Autodesk Inventor part; units mm, degrees
ref_plane "YZ Plane" through (0, 0, 0) normal (1, 0, 0) x (0, 1, 0)
ref_plane "XZ Plane" through (0, 0, 0) normal (0, 1, 0) x (-1, 0, 0)
ref_plane "XY Plane" through (0, 0, 0) normal (0, 0, 1) x (1, 0, 0)
sketch "스케치3" plane through (0, 0, 0) normal (0, 1, 0) x (-1, 0, 0)
  line L0 (34.9919, -14.4941) -> (14.4941, -34.9919)
  line L1 (14.4941, -34.9919) -> (-14.4941, -34.9919)
  line L2 (-14.4941, -34.9919) -> (-34.9919, -14.4941)
  line L3 (-34.9919, -14.4941) -> (-34.9919, 14.4941)
  line L4 (-34.9919, 14.4941) -> (-14.4941, 34.9919)
  line L5 (-14.4941, 34.9919) -> (14.4941, 34.9919)
  line L6 (14.4941, 34.9919) -> (34.9919, 14.4941)
  line L7 (34.9919, 14.4941) -> (34.9919, -14.4941)
  line L8 (32.5919, -13.5) -> (13.5, -32.5919)
  line L9 (13.5, -32.5919) -> (-13.5, -32.5919)
  line L10 (-13.5, -32.5919) -> (-32.5919, -13.5)
  line L11 (-32.5919, -13.5) -> (-32.5919, 13.5)
  line L12 (-32.5919, 13.5) -> (-13.5, 32.5919)
  line L13 (-13.5, 32.5919) -> (13.5, 32.5919)
  line L14 (13.5, 32.5919) -> (32.5919, 13.5)
  line L15 (32.5919, 13.5) -> (32.5919, -13.5)
  point P0 (0, 0)
  point P1 (0, 0)
  point P2 (0, 0)
  point P3 (0, 0)
  dimension "d43" = 27
  dimension "d44" = 2.4
extrude "돌출2" add sketch "스케치3" along normal blind 3.4 contours L0 L1 L2 L3 L4 L5 L6 L7 | L8 L9 L10 L11 L12 L13 L14 L15
sketch "스케치4" plane through (0, 3.4, 0) normal (0, 1, 0) x (1, 0, 0)
  line L0 (13.5, -32.5919) -> (-13.5, -32.5919)
  line L1 (-13.5, -32.5919) -> (-32.5919, -13.5)
  line L2 (-32.5919, -13.5) -> (-32.5919, 13.5)
  line L3 (-32.5919, 13.5) -> (-13.5, 32.5919)
  line L4 (-13.5, 32.5919) -> (13.5, 32.5919)
  line L5 (13.5, 32.5919) -> (32.5919, 13.5)
  line L6 (32.5919, 13.5) -> (32.5919, -13.5)
  line L7 (32.5919, -13.5) -> (13.5, -32.5919)
  line L8 (-13.9971, 33.7919) -> (13.9971, 33.7919)
  line L9 (13.9971, 33.7919) -> (33.7919, 13.9971)
  line L10 (33.7919, 13.9971) -> (33.7919, -13.9971)
  line L11 (33.7919, -13.9971) -> (13.9971, -33.7919)
  line L12 (13.9971, -33.7919) -> (-13.9971, -33.7919)
  line L13 (-13.9971, -33.7919) -> (-33.7919, -13.9971)
  line L14 (-33.7919, -13.9971) -> (-33.7919, 13.9971)
  line L15 (-33.7919, 13.9971) -> (-13.9971, 33.7919)
  line L16 (-13.1686, 31.7919) -> (13.1686, 31.7919)
  line L17 (13.1686, 31.7919) -> (31.7919, 13.1686)
  line L18 (31.7919, 13.1686) -> (31.7919, -13.1686)
  line L19 (31.7919, -13.1686) -> (13.1686, -31.7919)
  line L20 (13.1686, -31.7919) -> (-13.1686, -31.7919)
  line L21 (-13.1686, -31.7919) -> (-31.7919, -13.1686)
  line L22 (-31.7919, -13.1686) -> (-31.7919, 13.1686)
  line L23 (-31.7919, 13.1686) -> (-13.1686, 31.7919)
  point P0 (0, 0)
  point P1 (0, 0)
  point P2 (0, 0)
  point P3 (0, 0)
  dimension "d7" = 27
  dimension "d42" = 1.2
  dimension "d45" = 0.8
extrude "돌출3" cut sketch "스케치4" against normal blind 1.2 contours L0 L1 L2 L3 L4 L5 L6 L7 | L8 L9 L10 L11 L12 L13 L14 L15 | L16 L17 L18 L19 L20 L21 L22 L23
sketch "스케치5" plane through (0, 0, 0) normal (0, -1, 0) x (1, 0, 0)
  line L0 (10, 2.5) -> (20, 2.5)
  line L1 (20, 2.5) -> (20, -2.5)
  line L2 (20, -2.5) -> (10, -2.5)
  line L3 (10, -2.5) -> (10, 2.5)
  line L4 (10, 2.5) -> (20, -2.5) construction
  line L5 (20, 2.5) -> (10, -2.5) construction
  line L6 (-20, 2.5) -> (-10, 2.5)
  line L7 (-10, 2.5) -> (-10, -2.5)
  line L8 (-10, -2.5) -> (-20, -2.5)
  line L9 (-20, -2.5) -> (-20, 2.5)
  line L10 (-20, 2.5) -> (-10, -2.5) construction
  line L11 (-10, 2.5) -> (-20, -2.5) construction
  point P0 (0, 0)
  point P1 (15, 0)
  point P2 (-15, 0)
  dimension "d11" = 10
  dimension "d12" = 5
  dimension "d13" = 10
  dimension "d16" = 30
extrude "돌출4" add sketch "스케치5" along normal blind 10
sketch "스케치6" plane through (-10, 0, -2.5) normal (0, 0, -1) x (-1, 0, 0)
  circle A0 centre (5, -10) radius 5
  circle A1 centre (-25, -10) radius 5
  line L0 (-20, -10) -> (-30, -10)
  line L1 (10, -10) -> (0, -10)
  point P0 (-10, 0)
  dimension "d23" = 10
  dimension "d24" = 10
extrude "돌출5" add sketch "스케치6" against normal blind 5
sketch "스케치7" plane through (-10, 0, -2.5) normal (0, 0, -1) x (-1, 0, 0)
  circle A0 centre (5, -10) radius 1.25
  line L0 (10, 0) -> (10, -10)
  line L1 (0, 0) -> (10, 0)
  line L2 (4.7788, 0) -> (0, 0)
  circle A1 centre (-25, -10) radius 1.25
  point P0 (-10, 0)
  dimension "d27" = 2.5
  dimension "d28" = 5
  dimension "d31" = 30
extrude "돌출6" cut sketch "스케치7" against normal blind 5
sketch "스케치8" plane through (0, 0, 0) normal (0, -1, 0) x (1, 0, 0)
  circle A0 centre (0, -17.3205) radius 1.25
  line L0 (-10, 2.5) -> (-10, -2.5)
  point P0 (0, 0)
  point P1 (-10, 0)
  dimension "d38" = 2.5
  dimension "d39" = 17.3205
extrude "돌출7" cut sketch "스케치8" against normal blind 5
sketch "스케치9" plane through (0, 2.2, 0) normal (0, 1, 0) x (1, 0, 0)
  line L0 (-13.1686, 31.7919) -> (13.1686, 31.7919)
  line L1 (13.1686, 31.7919) -> (31.7919, 13.1686)
  line L2 (31.7919, 13.1686) -> (31.7919, -13.1686)
  line L3 (31.7919, -13.1686) -> (13.1686, -31.7919)
  line L4 (13.1686, -31.7919) -> (-13.1686, -31.7919)
  line L5 (-13.1686, -31.7919) -> (-31.7919, -13.1686)
  line L6 (-31.7919, -13.1686) -> (-31.7919, 13.1686)
  line L7 (-31.7919, 13.1686) -> (-13.1686, 31.7919)
  line L8 (-13.9971, 33.7919) -> (13.9971, 33.7919)
  line L9 (-12.6716, 30.5919) -> (12.6716, 30.5919)
  line L10 (12.6716, 30.5919) -> (30.5919, 12.6716)
  line L11 (30.5919, 12.6716) -> (30.5919, -12.6716)
  line L12 (30.5919, -12.6716) -> (12.6716, -30.5919)
  line L13 (12.6716, -30.5919) -> (-12.6716, -30.5919)
  line L14 (-12.6716, -30.5919) -> (-30.5919, -12.6716)
  line L15 (-30.5919, -12.6716) -> (-30.5919, 12.6716)
  line L16 (-30.5919, 12.6716) -> (-12.6716, 30.5919)
  point P0 (0, 0)
  point P1 (0, 0)
  point P2 (0, 0)
  dimension "d46" = 2
  dimension "d47" = 1.2
extrude "돌출8" add sketch "스케치9" along normal blind 0.6
properties part number "팔각형 OV-PAM 5패턴 상단 - 틈 너비 수정"
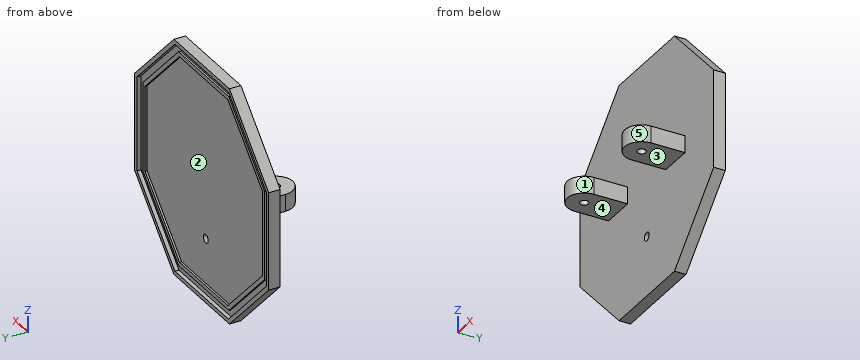
Here's how the part is built. I have some questions about the finished solid (model axes, mm). Face numbers are marked on the shaded views. A direction names the side the tool comes from. Round coordinates to 2 decimals unless told otherwise and drop trailing zeros. Loops run counter-clockwise (first coordinate to the right, second up) from the corner with the lowest first, then second, coordinate; pieces in that order, holes last.
1. Which directions (+Z, -Z, +X, -X, +Y, -Y) give clear straight access to the entire face, cutting with the end or side of a thin tool? Please do the marked faces 1, 2 and 3.
Answer list:
face 1: +Z, -Z, -Y
face 2: +Y
face 3: -Z, +X, -X, -Y
2. If we section it at C-C on x = 11: Write out the boundary of the cut face in (y, z).
Answer list:
outline: (-13, -2.5) - (0, -2.5) - (0, -34.99) - (3.4, -34.99) - (3.4, -33.79) - (2.2, -33.79) - (2.2, -31.79) - (2.8, -31.79) - (2.8, -30.59) - (2.2, -30.59) - (2.2, 30.59) - (2.8, 30.59) - (2.8, 31.79) - (2.2, 31.79) - (2.2, 33.79) - (3.4, 33.79) - (3.4, 34.99) - (0, 34.99) - (0, 2.5) - (-13, 2.5) - close
3. If we section it at B-B on x = 0: Write out the boundary of the cut face in (y, z).
Answer list:
outline: (0, -34.99) - (3.4, -34.99) - (3.4, -33.79) - (2.2, -33.79) - (2.2, -31.79) - (2.8, -31.79) - (2.8, -30.59) - (2.2, -30.59) - (2.2, -18.57) - (0, -18.57) - close; (0, -16.07) - (2.2, -16.07) - (2.2, 30.59) - (2.8, 30.59) - (2.8, 31.79) - (2.2, 31.79) - (2.2, 33.79) - (3.4, 33.79) - (3.4, 34.99) - (0, 34.99) - close
4. If we section it at D-D on z = 6.5: Write out the boundary of the cut face in (x, y), plus the area to 3 significant figures.
Answer list:
outline: (-34.99, 0) - (34.99, 0) - (34.99, 3.4) - (33.79, 3.4) - (33.79, 2.2) - (31.79, 2.2) - (31.79, 2.8) - (30.59, 2.8) - (30.59, 2.2) - (-30.59, 2.2) - (-30.59, 2.8) - (-31.79, 2.8) - (-31.79, 2.2) - (-33.79, 2.2) - (-33.79, 3.4) - (-34.99, 3.4) - close
area: 158 mm2
5. We'd pull the mould along X, two halves only. Please class the marked faces 4 and 5: +X half, -X half, draft (parallel to the pull), parting line (faces both ways), or undercut.
Answer list:
face 4: draft
face 5: undercut
6. If we section it at A-A on y = -7: Write out the boundary of the cut face in (x, z).
Answer list:
outline: (-20, -2.5) - (-10, -2.5) - (-10, 2.5) - (-20, 2.5) - close; (10, -2.5) - (20, -2.5) - (20, 2.5) - (10, 2.5) - close
7. If I drill on line 1 along Z through (x, y) = (-6, 2.75); line 2 along Y through (x, z) = (15, 1), over which ranges is the centre line in solid material (lowest first)?
Answer list:
line 1: z = -34.99 to -33.79, -31.79 to -30.59, 30.59 to 31.79, 33.79 to 34.99
line 2: y = -15 to -11.25, -8.75 to 2.2
8. For P1, Ø10, axis at y = -2.5, z = -12, coming from the +X side; P2, Ø3, axis at y = -9, z = 2.5, coming from the -X side; P3, Ø5.5, axis at y = -4, z = 1, coming from the +X side; P4, Ø20.5, axis at x = 8, z = 4, coming from the +Y side, each with a flat end and sliding along its axis, tell me the tip position at first contact or that it passes through.
Answer list:
P1: stops at x = 34.99
P2: stops at x = -20
P3: stops at x = 20
P4: stops at y = 2.2
